```python
from build123d import *

# Parameters (mm, degrees)
EXTRUDE1_DEPTH = 2
SKETCH3_R      = 4
SKETCH3_R_2    = 1.85
EXTRUDE2_DEPTH = 2


with BuildPart() as part:
    # Sketch2 → Extrude1 (new body)
    with BuildSketch(Plane(origin=(0, 0, 0), x_dir=(1, 0, 0), z_dir=(0, 1, 0))):
        with BuildLine():
            Line((-13.5, -32), (-13.5, 32))
            ThreePointArc((-13.5, 32), (0, 45.5), (13.5, 32))
            Line((13.5, 32), (13.5, -32))
            ThreePointArc((13.5, -32), (0, -45.5), (-13.5, -32))
        make_face()
    extrude(amount=EXTRUDE1_DEPTH)

    # Sketch3 → Extrude2 (cut)
    with BuildSketch(Plane(origin=(0, 2, 0), x_dir=(1, 0, 0), z_dir=(0, 1, 0))):
        with Locations((0, -16)):
            Circle(SKETCH3_R)
        with Locations((0, 16)):
            Circle(SKETCH3_R)
        Circle(SKETCH3_R)
        with Locations((0, 8)):
            Circle(SKETCH3_R_2)
        with Locations((0, -8)):
            Circle(SKETCH3_R_2)
        with Locations((8, 0)):
            Circle(SKETCH3_R_2)
        with Locations((-8, 0)):
            Circle(SKETCH3_R_2)
        with Locations((0, -24)):
            Circle(SKETCH3_R_2)
        with Locations((8, -32)):
            Circle(SKETCH3_R_2)
        with Locations((0, -32)):
            Circle(SKETCH3_R)
        with Locations((-8, -32)):
            Circle(SKETCH3_R_2)
        with Locations((-5.66, -37.66)):
            Circle(SKETCH3_R_2)
        with Locations((5.66, -37.66)):
            Circle(SKETCH3_R_2)
        with Locations((0, -40)):
            Circle(SKETCH3_R_2)
        with Locations((-5.66, -26.34)):
            Circle(SKETCH3_R_2)
        with Locations((5.66, -26.34)):
            Circle(SKETCH3_R_2)
        with Locations((0, 40)):
            Circle(SKETCH3_R_2)
        with Locations((8, 32)):
            Circle(SKETCH3_R_2)
        with Locations((0, 32)):
            Circle(SKETCH3_R)
        with Locations((-8, 32)):
            Circle(SKETCH3_R_2)
        with Locations((-5.66, 26.34)):
            Circle(SKETCH3_R_2)
        with Locations((5.66, 26.34)):
            Circle(SKETCH3_R_2)
        with Locations((0, 24)):
            Circle(SKETCH3_R_2)
        with Locations((-5.66, 37.66)):
            Circle(SKETCH3_R_2)
        with Locations((5.66, 37.66)):
            Circle(SKETCH3_R_2)
    extrude(amount=-EXTRUDE2_DEPTH, mode=Mode.SUBTRACT)


solid = part.part
```
Source: CAD feature listing. Evaluate the final solid. Frame: model axes, mm. Round coordinates to 2 decimals unless told otherwise and drop trailing zeros. Loops run counter-clockwise (first coordinate to the right, second up) from the corner with the lowest first, then second, coordinate; pieces in that order, holes last. Notation, with made-up numbers: M -2,78 L 48,78 A19 cw 48,111 Z; hole C 74,-23.75 d6. An arc over 180 degrees is marked long. Use a Markdown table: item, result. Add a question column.
1. Section query D-D on x = 5.25. Return the cut outline in (y, z), then the cut area to 3 significant figures.
2. Section query A-A on z = -16. Return the cut outline in (x, y), then the cut area to 3 significant figures.
3. Line query: line 1 (X direction, y = 0.6, z = -32); line 2 (Z direction, x = -5, y = 0.5); line 3 (Z direction, x = -6, y = 1.15). Output: solid intervals per line, ascending.
4. Contact query for flat-ended pins moving along their axis: P1, Ø5, axis at x = 0, z = -8, coming from the -Y side; P2, Ø3, axis at x = 0, z = -24, coming from the -Y side. Output: stop coordinate, or through.
5. Mould query, pull axis X, two halves, no side actions, for faces 1 (the flat face through (-6, 0, -1)), 2 (the cylindrical face through (6.636, 1.014, -33.25)), 3 (the cylindrical face through (-0.297, 0.986, -45.497)). Classes: pulls with the +X half, pulls with the -X half, needs draft (parallel to the pull), parting line crosses it, or undercut.
6. Section query C-C on z = 0. Return the cut outline in (x, y), then the cut area to 3 significant figures.
7. Section query B-B on y = 1.05. Give the number of separate pieces and of enclosed holes in the cut face, then the cut area to 3 significant figures.
Reported:
| question | item | result |
|---|---|---|
| 1 | outline | M 0,-44.44 L 2,-44.44 L 2,-39.46 L 0,-39.46 Z; M 0,-35.86 L 2,-35.86 L 2,-28.14 L 0,-28.14 Z; M 0,-24.54 L 2,-24.54 L 2,24.54 L 0,24.54 Z; M 0,28.14 L 2,28.14 L 2,35.86 L 0,35.86 Z; M 0,39.46 L 2,39.46 L 2,44.44 L 0,44.44 Z |
| 1 | area | 149 mm² |
| 2 | outline | M -13.5,0 L -4,0 L -4,2 L -13.5,2 Z; M 4,0 L 13.5,0 L 13.5,2 L 4,2 Z |
| 2 | area | 38.0 mm² |
| 3 | line 1 | x = -13.5 to -9.85, -6.15 to -4, 4 to 6.15, 9.85 to 13.5 |
| 3 | line 2 | z = -44.54 to -39.39, -35.93 to -28.07, -24.61 to 24.61, 28.07 to 35.93, 39.39 to 44.54 |
| 3 | line 3 | z = -44.09 to -39.48, -35.84 to -28.16, -24.52 to 24.52, 28.16 to 35.84, 39.48 to 44.09 |
| 4 | P1 | stops at y = 0 |
| 4 | P2 | passes through |
| 5 | face 1 | needs draft |
| 5 | face 2 | undercut |
| 5 | face 3 | parting line crosses it |
| 6 | outline | M -13.5,0 L -9.85,0 L -9.85,2 L -13.5,2 Z; M -6.15,0 L -4,0 L -4,2 L -6.15,2 Z; M 4,0 L 6.15,0 L 6.15,2 L 4,2 Z; M 9.85,0 L 13.5,0 L 13.5,2 L 9.85,2 Z |
| 6 | area | 23.2 mm² |
| 7 | separate pieces | 1 |
| 7 | enclosed holes | 25 |
| 7 | area | 1,830 mm² |
